Here's how the part is built. I have some questions about the finished solid (model axes, mm). A direction names the side the tool comes from. Coordinates: 2 decimals unless noted, no trailing zeros. Order: outer loops, then holes, each group sorted by start corner. A loop starts at its lowest first (then second) coordinate and runs counter-clockwise, first axis right, second up. Notation, with made-up numbers: M 61.25,71.25 L 85.25,71.25 A16 ccw 85.25,75.25 Z; hole C 16.25,25 d5. An arc over 180 degrees is marked long. Answer as CSV lines item,"result". Start each with the question number.
Autodesk Inventor part; units mm, degrees
ref_plane "Начальная плоскость" through (0, 0, -32.5) normal (0, 0, 1) x (1, 0, 0)
ref_plane "Конечная плоскость" through (0, 0, 250) normal (0, 0, 1) x (1, 0, 0)
ref_plane "РабПлоскость8" through (18, -177.5, -32.5) normal (0, 0, -1) x (-1, 0, 0)
ref_plane "Начальная плоскость" through (0, 0, -32.5) normal (0, 0, 1) x (1, 0, 0)
ref_plane "Конечная плоскость" through (0, 0, 250) normal (0, 0, 1) x (1, 0, 0)
sketch "Эскиз" plane through (0, 0, 0) normal (0, 0, 1) x (1, 0, 0)
  line L0 (36, -32.5) -> (0, -32.5)
  line L1 (36, -32.5) -> (36, -28.696)
  line L2 (33.6994, -26.2039) -> (9.9215, -24.3017)
  line L3 (4.4, -18.3208) -> (4.4, 18.3208)
  line L4 (33.6994, 26.2039) -> (9.9215, 24.3017)
  line L5 (36, 28.696) -> (36, 32.5)
  line L6 (0, 32.5) -> (36, 32.5)
  line L7 (0, -32.5) -> (0, 32.5)
  arc A0 (4.4, -18.3208) -> (9.9215, -24.3017) centre (10.4, -18.3208) ccw
  arc A1 (9.9215, 24.3017) -> (4.4, 18.3208) centre (10.4, 18.3208) ccw
  arc A2 (36, -28.696) -> (33.6994, -26.2039) centre (33.5, -28.696) ccw
  arc A3 (33.6994, 26.2039) -> (36, 28.696) centre (33.5, 28.696) ccw
  line L8 (0, 45.5) -> (0, -45.5) construction
  line L9 (-7.2974, 0) -> (43.7847, 0) construction
  point P0 (36, -26.388)
  point P1 (4.4, -23.86)
  point P2 (4.4, 23.86)
  point P3 (36, 26.388)
  dimension "d3" = 36
  dimension "d5" = 4.4
  dimension "d7" = 65
  dimension "d9" = 8.64
  dimension "d11" = 8.64
  dimension "d13" = 6.112
  dimension "d15" = 6.112
  dimension "d22" = 6
  dimension "d23" = 2.5
  dimension "d24" = 32.5
  dimension "d25" = 0
extrude "Тело" add sketch "Эскиз" along normal up to surface (282.5 mm away) from surface at -32.5
sketch "Sketch3" plane through (0, 0, 0) normal (0, 0, 1) x (1, 0, 0)
  line L0 (0, 0) -> (10, 0)
ref_plane "Work Plane7" through (0, 0, 0) normal (0, -1, 0) x (1, 0, 0)
sketch "Sketch4" plane through (0, 0, 0) normal (0, -1, 0) x (1, 0, 0)
  line L0 (-2, -32.5) -> (12, -32.5)
  line L1 (-2, 250) -> (12, 250)
  dimension "d29" = 282.5
ref_plane "РабПлоскость8" through (18, -177.5, -32.5) normal (0, 0, -1) x (-1, 0, 0)
split "Разделение1" plane through (18, -177.5, -32.5) removes the side toward (0, 0, -1)
equation "\"d3\" = b"
equation "\"d7\" = ParH"
equation "\"d22\" = R"
equation "\"d23\" = R1"
equation "\"d24\" = 0.5 * d7"
equation "\"d16\" = G_L"
equation "\"R1\" = 2.5"
equation "\"R\" = 6"
equation "\"t1\" = 4.4"
equation "\"t2\" = 7.2"
equation "\"ParH\" = 65"
equation "\"b\" = 36"
equation "\"msp_x1\" = 0.04 * b"
equation "\"msp_x2\" = -0.08 * t1 + 0.04 * b"
equation "\"G_L\" = d29"
equation "\"ex\" = 0"
equation "\"G_OFFSET_START\" = 32.5"
equation "\"G_OFFSET_END\" = 0"
equation "\"d26\" = -G_OFFSET_START"
properties part number "Швеллер 6.5U-282,5 ГОСТ 8240-97"
1) Suppose I cut it at A-A on x = 7. Please give me the cut outline in (y, z), plus the area to 3 significant figures.
2) Suppose I cut it at B-B on z = 45. Please give me the cut outline in (x, y).
3) Suppose I cut it at D-D on x = 20. Please give me the cut outline in (y, z).
4) If we mould it in two halves opening along Y, with no side actions, what happens to faces 1 (the face through (3, 0, -32.5)), 2 (the face through (21.977, 25.266, 106.773)), 3 (the face through (18, -32.5, 107)), 4 (the face through (18, 32.5, 107))? For each: released by +Y, released by -Y, zero draft, split by the parting line, or undercut.
5) I need wall thicknesses on line 1 (X direction, y = 12.5, z = 22); line 2 (Y direction, x = 9.5, z = 25.5); line 3 (Y direction, x = 13.5, z = 142.5). Which ranges of each line are inside material? Lowest first, please. Write a range as [from, to].
6) Which directions (+Z, -Z, +X, -X, +Y, -Y) give clear straight access to the entire face, cutting with the end or side of a thin tool? Please do faces 5 (the face through (4.4, 0, 107)), 6 (the face through (0, 0, 107)).
7) Suppose I cut it at C-C on y = -7.5. Please give me the cut outline in (x, z).
8) Will these pins go through, and if not, where does the flat tip stop? pin 1 Ø12 at (x, y) = (28.5, 16.5) entering from -Z; pin 2 Ø11 at (y, z) = (-6.5, 87.5) entering from +X; pin 3 Ø1 at (y, z) = (22, 6.5) entering from +X.
Output:
1,outline,"M -32.5,-32.5 L -23.26,-32.5 L -23.26,250 L -32.5,250 Z; M 23.26,-32.5 L 32.5,-32.5 L 32.5,250 L 23.26,250 Z"
1,area,"5,220 mm²"
2,outline,"M 0,-32.5 L 36,-32.5 L 36,-28.7 A2.5 ccw 33.7,-26.2 L 9.92,-24.3 A6 cw 4.4,-18.32 L 4.4,18.32 A6 cw 9.92,24.3 L 33.7,26.2 A2.5 ccw 36,28.7 L 36,32.5 L 0,32.5 Z"
3,outline,"M -32.5,-32.5 L -25.11,-32.5 L -25.11,250 L -32.5,250 Z; M 25.11,-32.5 L 32.5,-32.5 L 32.5,250 L 25.11,250 Z"
4,face 1,"zero draft"
4,face 2,"undercut"
4,face 3,"released by -Y"
4,face 4,"released by +Y"
5,line 1,"[0, 4.4]"
5,line 2,"[-32.5, -24.25], [24.25, 32.5]"
5,line 3,"[-32.5, -24.59], [24.59, 32.5]"
6,face 5,"+Z, -Z, +X"
6,face 6,"+Z, -Z, -X, +Y, -Y"
7,outline,"M 0,-32.5 L 4.4,-32.5 L 4.4,250 L 0,250 Z"
8,pin 1,"through"
8,pin 2,"x = 4.4"
8,pin 3,"x = 6.09"
